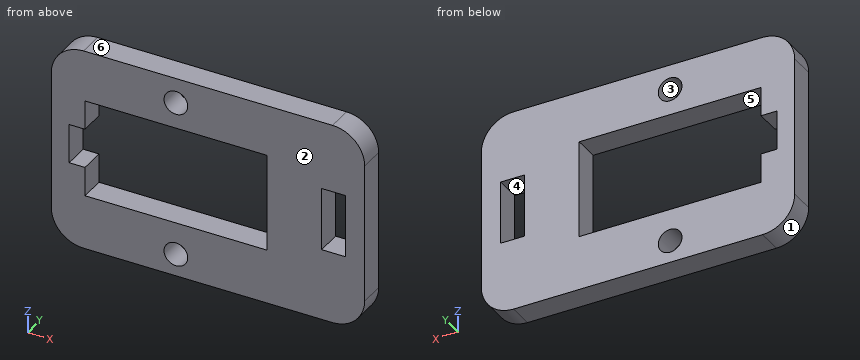
```python
from build123d import *

# Parameters (mm, degrees)
SKETCH1_R           = 1.4972665
SKETCH1_W           = 2.994723397
SKETCH1_H           = 8.000362859
BOSS_EXTRUDE1_DEPTH = 3.175


with BuildPart() as part:
    # Sketch1 → Boss-Extrude1 (new body)
    with BuildSketch(Plane(origin=(0, 0, 0), x_dir=(1, 0, 0), z_dir=(0, 1, 0))):
        with BuildLine():
            Line((-15.724689345, 13.36466939), (15.717340342, 13.36466939))
            ThreePointArc((15.717340342, 13.36466939), (18.593486483, 12.173330652), (19.784825221, 9.297184512))
            Line((19.784825221, 9.297184512), (19.784825221, -8.374175229))
            ThreePointArc((19.784825221, -8.374175229), (18.595583797, -11.245258003), (15.724501023, -12.434499427))
            Line((15.724501023, -12.434499427), (-15.717328779, -12.434499427))
            ThreePointArc((-15.717328779, -12.434499427), (-18.593478625, -11.243159154), (-19.784818899, -8.367009308))
            Line((-19.784818899, -8.367009308), (-19.784818899, 9.304539837))
            ThreePointArc((-19.784818899, 9.304539837), (-18.595634485, 12.175484977), (-15.724689345, 13.36466939))
        make_face()
        with Locations(Location((-4.054054374, 10.549054746, 0), (0, 0, 270))):
            Circle(SKETCH1_R, mode=Mode.SUBTRACT)
        with Locations(Location((-4.054054375, -9.251582203, 0), (0, 0, 270))):
            Circle(SKETCH1_R, mode=Mode.SUBTRACT)
        Polygon((-15.533671416, 6.449054402), (7.425689399, 6.449054402), (7.425689399, -5.951480927), (-15.533671416, -5.951480927), (-15.533671416, -2.251386169), (-17.530124434, -2.251386169), (-17.530124434, 2.748832682), (-15.533671416, 2.748832682), align=None, mode=Mode.SUBTRACT)
        with Locations((15.846212781, 0.248720813)):
            Rectangle(SKETCH1_W, SKETCH1_H, mode=Mode.SUBTRACT)
    extrude(amount=BOSS_EXTRUDE1_DEPTH)


solid = part.part
```
Could you check a few things on this model? Use its own coordinates, in mm. Face numbers are marked on the shaded views. A direction names the side the tool comes from. Round coordinates to 2 decimals unless told otherwise and drop trailing zeros. Order: outer loops, then holes, each group sorted by start corner. A loop starts at its lowest first (then second) coordinate and runs counter-clockwise, first axis right, second up. Notation, with made-up numbers: M 57.5,7.25 L 115.5,7.25 A25 cw 115.5,31.25 Z; hole C 80,63 d7. An arc over 180 degrees is marked long. One line per question, with ' | ' between items. Start each with the question number.
(1) Suppose I cut it at D-D on y = 1.15. List the corners of the cut face in (x, z) for me.
(2) Suppose I cut it at B-B on x = -8. List the corners of the cut face in (y, z) for me (1 decimal).
(3) For the marked faces 5 and 6, which set-ups out of +Z, -Z, +X, -X, +Y, -Y let a thin tool reach every point of the face, with its end or its side?
(4) Please list where these lines run through material, in increasing order: line 1 along X through (y, z) = (1.25, 1.25); line 2 along Z through (x, y) = (-4, 1); line 3 along Z through (x, y) = (16, 1.4).
(5) For P1, Ø1, axis at x = -17, y = 2, coming from the +Z side, with a flat end and sliding along its axis, tell me the tip position at first contact or that it passes through.
(6) Suppose I cut it at C-C on z = -1. List the corners of the cut face in (x, y) for me (3 decimals).
(7) Suppose I cut it at A-A on z = -5.75. List the corners of the cut face in (x, y) for me (3 decimals).
(8) Thinking about a two-plate mould opening in Z: for the marked faces 1, 2, 3 and 4, which applies, +Z half, -Z half, draft (parallel to the pull), parting line (faces both ways), or undercut?
Geometry results:
1) outline: M -19.78,-9.3 A4.06 ccw -15.72,-13.36 L 15.72,-13.36 A4.07 ccw 19.78,-9.3 L 19.78,8.37 A4.06 ccw 15.72,12.43 L -15.72,12.43 A4.07 ccw -19.78,8.37 Z; hole M -17.53,-2.75 L -15.53,-2.75 L -15.53,-6.45 L 7.43,-6.45 L 7.43,5.95 L -15.53,5.95 L -15.53,2.25 L -17.53,2.25 Z; hole C -4.05,-10.55 d2.99; hole C -4.05,9.25 d2.99; hole M 14.35,-4.25 L 17.34,-4.25 L 17.34,3.75 L 14.35,3.75 Z
2) outline: M 0,-13.4 L 3.2,-13.4 L 3.2,-6.4 L 0,-6.4 Z; M 0,6 L 3.2,6 L 3.2,12.4 L 0,12.4 Z
3) face 5: +Y, -Y | face 6: +Z, +X, -X, +Y, -Y
4) line 1: -19.78 to -17.53, 7.43 to 14.35, 17.34 to 19.78 | line 2: -13.36 to -12.05, -9.05 to -6.45, 5.95 to 7.76, 10.75 to 12.43 | line 3: -13.35 to -4.25, 3.75 to 12.43
5) P1: z = 12.36
6) outline: M -19.785,0 L -17.53,0 L -17.53,3.175 L -19.785,3.175 Z; M 7.426,0 L 14.349,0 L 14.349,3.175 L 7.426,3.175 Z; M 17.344,0 L 19.785,0 L 19.785,3.175 L 17.344,3.175 Z
7) outline: M -19.785,0 L -15.534,0 L -15.534,3.175 L -19.785,3.175 Z; M 7.426,0 L 19.785,0 L 19.785,3.175 L 7.426,3.175 Z
8) face 1: -Z half | face 2: draft | face 3: undercut | face 4: undercut
